from build123d import *

# Parameters (mm, degrees)
SKETCH3_R           = 37.5
SKETCH3_R_2         = 32.5
BOSS_EXTRUDE1_DEPTH = 30
SKETCH4_R           = 50
BOSS_EXTRUDE2_DEPTH = 5
SKETCH5_W           = 65
SKETCH5_H           = 8.049170271
BOSS_EXTRUDE3_DEPTH = 65
FILLET1_R           = 25
SKETCH6_R           = 15
CUT_EXTRUDE1_DEPTH  = 10


with BuildPart() as part:
    # Sketch3 → Boss-Extrude1 (new body)
    with BuildSketch(Plane(origin=(0, 0, 0), x_dir=(1, 0, 0), z_dir=(0, 1, 0))):
        with Locations(Location((0, 0, 0), (0, 0, 270))):
            Circle(SKETCH3_R)
        with Locations(Location((0, 0, 0), (0, 0, 270))):
            Circle(SKETCH3_R_2, mode=Mode.SUBTRACT)
    extrude(amount=BOSS_EXTRUDE1_DEPTH)

    # Sketch4 → Boss-Extrude2 (add)
    with BuildSketch(Plane(origin=(0, 30, 0), x_dir=(1, 0, 0), z_dir=(0, 1, 0))):
        with Locations(Location((0, 0, 0), (0, 0, 270))):
            Circle(SKETCH4_R)
    extrude(amount=BOSS_EXTRUDE2_DEPTH)

    # Sketch5 → Boss-Extrude3 (add)
    with BuildSketch(Plane(origin=(0, 35, 0), x_dir=(1, 0, 0), z_dir=(0, 1, 0))):
        with Locations((0, -22.269371084)):
            Rectangle(SKETCH5_W, SKETCH5_H)
    extrude(amount=BOSS_EXTRUDE3_DEPTH)

    # Fillet1
    fillet1_edges = [part.edges().sort_by_distance(p)[0] for p in [
        (-32.5, 100, 22.269371084),
        (32.5, 100, 22.269371084),
    ]]
    fillet(fillet1_edges, radius=FILLET1_R)

    # Sketch6 → Cut-Extrude1 (cut)
    with BuildSketch(Plane(origin=(0, 0, 18.244785948), x_dir=(-1, 0, 0), z_dir=(0, 0, -1))):
        with Locations((0, 75.757344868)):
            Circle(SKETCH6_R)
    extrude(amount=-CUT_EXTRUDE1_DEPTH, mode=Mode.SUBTRACT)


solid = part.part
Can you work these out from the model? Positions are in its coordinate system, mm. A direction names the side the tool comes from. Coordinates: 2 decimals unless noted, no trailing zeros. Write each loop counter-clockwise with the first axis right and the second up, starting at its lowest first coordinate (ties: lowest second). Pieces come first, ordered by that corner, then holes.
Q1. Please list where these lines run through material, in increasing order: L1, parallel to Y at x = 0, z = 20; L2, parallel to X at y = 17.5, z = 0; L3, parallel to Y at x = 30, z = -11.5.
Results found:
L1: y = 30 to 60.76, 90.76 to 100
L2: x = -37.5 to -32.5, 32.5 to 37.5
L3: y = 30 to 35
Q2. If we mould it in two halves opening along X, with no side actions, what happens to faces 1 (the face through (-22.818, 14.79, -29.759)), 2 (the face through (0, 100, 22)), 3 (the face through (1.95, 90.63, 22.21))? For each: +X half, -X half, draft (parallel to the pull), parting line (faces both ways), or undercut.
Results found:
face 1: parting line
face 2: draft
face 3: undercut
Q3. Imagine slicing it at B-B, the plane y = 84. List the corners of the cut face in (x, z) for me.
Results found:
outline: (-30.82, 18.24) - (-12.53, 18.24) - (-12.53, 26.29) - (-30.82, 26.29) - close; (12.53, 18.24) - (30.82, 18.24) - (30.82, 26.29) - (12.53, 26.29) - close
Q4. Imagine slicing it at A-A, the plane x = 0. List the corners of the cut face in (y, z) for me, plus the area to 3 significant figures.
Results found:
outline: (0, -37.5) - (30, -37.5) - (30, -50) - (35, -50) - (35, 18.24) - (60.76, 18.24) - (60.76, 26.29) - (35, 26.29) - (35, 50) - (30, 50) - (30, 37.5) - (0, 37.5) - (0, 32.5) - (30, 32.5) - (30, -32.5) - (0, -32.5) - close; (90.76, 18.24) - (100, 18.24) - (100, 26.29) - (90.76, 26.29) - close
area: 1,080 mm2
Q5. Imagine slicing it at D-D, the plane x = 17. List the corners of the cut face in (y, z) for me.
Results found:
outline: (0, -33.43) - (30, -33.43) - (30, -47.02) - (35, -47.02) - (35, 18.24) - (98.12, 18.24) - (98.12, 26.29) - (35, 26.29) - (35, 47.02) - (30, 47.02) - (30, 33.43) - (0, 33.43) - (0, 27.7) - (30, 27.7) - (30, -27.7) - (0, -27.7) - close
Q6. For P1, Ø9, axis at y = 46.5, z = 20.5, coming from the +X side; P2, Ø6.5, axis at y = 51.5, z = 22.5, coming from the -X side; P3, Ø19.5, axis at x = 5, y = 61.5, coming from the -Z side, each with a flat end and sliding along its axis, tell me the tip position at first contact or that it passes through.
Results found:
P1: stops at x = 32.5
P2: stops at x = -32.5
P3: stops at z = 18.24
Q7. Imagine slicing it at C-C, the plane z = 0. List the corners of the cut face in (x, y) for me.
Results found:
outline: (-50, 30) - (-37.5, 30) - (-37.5, 0) - (-32.5, 0) - (-32.5, 30) - (32.5, 30) - (32.5, 0) - (37.5, 0) - (37.5, 30) - (50, 30) - (50, 35) - (-50, 35) - close
Q8. Which directions (+Z, -Z, +X, -X, +Y, -Y) give clear straight access to the entire face, cutting with the end or side of a thin tool? Please do faces 4 (the face through (-32.5, 55, 22)), 5 (the face through (32.5, 55, 22)), 6 (the face through (37, 30, 7)).
Results found:
face 4: +Z, -Z, -X, +Y
face 5: +Z, -Z, +X, +Y
face 6: -Y
